Input: part model. Units: mm. Frame: model coordinates. A direction names the side the tool comes from. Coordinates: 2 decimals unless noted, no trailing zeros. Loops run counter-clockwise (first coordinate to the right, second up) from the corner with the lowest first, then second, coordinate; pieces in that order, holes last.
(1) Section C-C, the plane z = 7.5. Return loops of the section in (x, y).
(2) Section A-A, the plane x = 0. Return loops of the section in (y, z).
(3) Set-up query: faces 1 (the face through (-5.158, -3.955, 7.866)), 2 (the face through (0, -5, 1.25)). Return all of +Z, -Z, +X, -X, +Y, -Y with unobstructed straight access to the full face (end or side cutting, diameter ignored); none if empty.
(4) Contact query for flat-ended pins moving along their axis: P1, Ø4, axis at y = -4, z = 3, coming from the -X side; P2, Ø4, axis at x = 4.5, y = -2, coming from the -Z side; P3, Ø5, axis at x = -4.5, z = 4.5, coming from the +Y side; P4, Ø1, axis at x = 2, z = 1, coming from the +Y side. Output: stop coordinate, or through.
(5) Line query: L1, parallel to Y at x = 0, z = 6.75; L2, parallel to Z at x = -3.25, y = -3.5; L3, parallel to X at y = -0.5, z = 3.5. Output: solid intervals per line, ascending.
(6) Section D-D, the plane y = -2. Return loops of the section in (x, z).
(7) Mould query, pull axis Z, two halves, no side actions, for faces 3 (the face through (-5.158, -3.955, 0.616)), 4 (the face through (0, -5, 7.25)), 5 (the face through (2.192, -4.214, 4.208)), 6 (the face through (0, 2, 8.5)). Classes: released by +Z, released by -Z, zero draft, split by the parting line, or undercut.
```python
from build123d import *

# Parameters (mm, degrees)
SKETCH_1_R          = 6.5
EXTRUDE_1_DEPTH     = 1.25
SKETCH_2_R          = 4.75
EXTRUDE_2_DEPTH     = 6
SKETCH_3_R          = 6.5
EXTRUDE_3_DEPTH     = 1.25
SKETCH_4_R          = 1.5
CUT_EXTRUDE_1_DEPTH = 9.5


with BuildPart() as part:
    # 草图1 → 凸台-拉伸1 (new body)
    with BuildSketch(Plane.XY):
        Circle(SKETCH_1_R)
    extrude(amount=EXTRUDE_1_DEPTH)

    # 草图2 → 凸台-拉伸2 (add)
    with BuildSketch(Plane.XY.offset(1.25)):
        Circle(SKETCH_2_R)
    extrude(amount=EXTRUDE_2_DEPTH)

    # 草图3 → 凸台-拉伸3 (add)
    with BuildSketch(Plane.XY.offset(7.25)):
        Circle(SKETCH_3_R)
    extrude(amount=EXTRUDE_3_DEPTH)

    # 草图4 → 切除-拉伸1 (cut, through all)
    with BuildSketch(Plane(origin=(0, 0, 0), x_dir=(-1, 0, 0), z_dir=(0, 0, -1))):
        Circle(SKETCH_4_R)
    extrude(amount=-CUT_EXTRUDE_1_DEPTH, mode=Mode.SUBTRACT)


solid = part.part
```
Report:
1. outline: circle Ø13 at (0, 0); hole circle Ø3 at (0, 0)
2. outline: (-6.5, 0) - (-1.5, 0) - (-1.5, 8.5) - (-6.5, 8.5) - (-6.5, 7.25) - (-4.75, 7.25) - (-4.75, 1.25) - (-6.5, 1.25) - close; (1.5, 0) - (6.5, 0) - (6.5, 1.25) - (4.75, 1.25) - (4.75, 7.25) - (6.5, 7.25) - (6.5, 8.5) - (1.5, 8.5) - close
3. face 1: +Z, -Z
3. face 2: none
4. P1: stops at x = -5.75
4. P2: stops at z = 0
4. P3: stops at y = 4.31
4. P4: stops at y = 6.32
5. L1: y = -4.75 to -1.5, 1.5 to 4.75
5. L2: z = 0 to 1.25, 7.25 to 8.5
5. L3: x = -4.72 to -1.41, 1.41 to 4.72
6. outline: (-6.18, 0) - (6.18, 0) - (6.18, 1.25) - (4.31, 1.25) - (4.31, 7.25) - (6.18, 7.25) - (6.18, 8.5) - (-6.18, 8.5) - (-6.18, 7.25) - (-4.31, 7.25) - (-4.31, 1.25) - (-6.18, 1.25) - close
7. face 3: zero draft
7. face 4: undercut
7. face 5: undercut
7. face 6: released by +Z
